Design review of the part built by this model. Coordinates are the model's own, in mm. Give positions to 0.01 mm unless a question says otherwise; leave off trailing zeros. Use CSV: the item, a comma, the result in double quotes.
from build123d import *

# Parameters (mm, degrees)
SKETCH2_W           = 3.175
SKETCH2_H           = 5.08
BOSS_EXTRUDE1_DEPTH = 3.175


with BuildPart() as part:
    # Sketch2 → Boss-Extrude1 (new body)
    with BuildSketch(Plane(origin=(0, 0, 0), x_dir=(1, 0, 0), z_dir=(0, 1, 0))):
        Polygon((-58.640729436, -170.164220965), (150.909270564, -170.164220965), (150.909270564, -134.604220965), (141.384270564, -134.604220965), (141.384270564, -129.524220965), (150.909270564, -129.524220965), (150.909270564, -93.964220965), (141.384270564, -93.964220965), (141.384270564, -88.884220965), (150.909270564, -88.884220965), (150.909270564, -43.164220965), (141.384270564, -43.164220965), (141.384270564, -38.084220965), (150.909270564, -38.084220965), (150.909270564, -2.524220965), (141.384270564, -2.524220965), (141.384270564, 2.555779035), (150.909270564, 2.555779035), (150.909270564, 39.385779035), (-58.640729436, 39.385779035), (-58.640729436, 2.555779035), (-49.115729436, 2.555779035), (-49.115729436, -2.524220965), (-58.640729436, -2.524220965), (-58.640729436, -38.084220965), (-49.115729436, -38.084220965), (-49.115729436, -43.164220965), (-58.640729436, -43.164220965), (-58.640729436, -88.884220965), (-49.115729436, -88.884220965), (-49.115729436, -93.964220965), (-58.640729436, -93.964220965), (-58.640729436, -129.524220965), (-49.115729436, -129.524220965), (-49.115729436, -134.604220965), (-58.640729436, -134.604220965), align=None)
        with Locations((-53.878229436, -162.544220965)):
            Rectangle(SKETCH2_W, SKETCH2_H, mode=Mode.SUBTRACT)
        with Locations((146.146770564, -162.544220965)):
            Rectangle(SKETCH2_W, SKETCH2_H, mode=Mode.SUBTRACT)
        with Locations((-53.878229436, -152.384220965)):
            Rectangle(SKETCH2_W, SKETCH2_H, mode=Mode.SUBTRACT)
        with Locations((-53.878229436, -142.224220965)):
            Rectangle(SKETCH2_W, SKETCH2_H, mode=Mode.SUBTRACT)
        with Locations((-53.878229436, -121.904220965)):
            Rectangle(SKETCH2_W, SKETCH2_H, mode=Mode.SUBTRACT)
        with Locations((-53.878229436, -111.744220965)):
            Rectangle(SKETCH2_W, SKETCH2_H, mode=Mode.SUBTRACT)
        with Locations((-53.878229436, -101.584220965)):
            Rectangle(SKETCH2_W, SKETCH2_H, mode=Mode.SUBTRACT)
        with Locations((-53.878229436, -81.264220965)):
            Rectangle(SKETCH2_W, SKETCH2_H, mode=Mode.SUBTRACT)
        with Locations((-53.878229436, -71.104220965)):
            Rectangle(SKETCH2_W, SKETCH2_H, mode=Mode.SUBTRACT)
        with Locations((-53.878229436, -60.944220965)):
            Rectangle(SKETCH2_W, SKETCH2_H, mode=Mode.SUBTRACT)
        with Locations((-53.878229436, -50.784220965)):
            Rectangle(SKETCH2_W, SKETCH2_H, mode=Mode.SUBTRACT)
        with Locations((-53.878229436, -30.464220965)):
            Rectangle(SKETCH2_W, SKETCH2_H, mode=Mode.SUBTRACT)
        with Locations((-53.878229436, -20.304220965)):
            Rectangle(SKETCH2_W, SKETCH2_H, mode=Mode.SUBTRACT)
        with Locations((-53.878229436, -10.144220965)):
            Rectangle(SKETCH2_W, SKETCH2_H, mode=Mode.SUBTRACT)
        with Locations((-53.878229436, 10.175779035)):
            Rectangle(SKETCH2_W, SKETCH2_H, mode=Mode.SUBTRACT)
        with Locations((-53.878229436, 20.335779035)):
            Rectangle(SKETCH2_W, SKETCH2_H, mode=Mode.SUBTRACT)
        with Locations((-53.878229436, 30.495779035)):
            Rectangle(SKETCH2_W, SKETCH2_H, mode=Mode.SUBTRACT)
        with Locations((146.146770564, 30.495779035)):
            Rectangle(SKETCH2_W, SKETCH2_H, mode=Mode.SUBTRACT)
        with Locations((146.146770564, 20.335779035)):
            Rectangle(SKETCH2_W, SKETCH2_H, mode=Mode.SUBTRACT)
        with Locations((146.146770564, 10.175779035)):
            Rectangle(SKETCH2_W, SKETCH2_H, mode=Mode.SUBTRACT)
        with Locations((146.146770564, -10.144220965)):
            Rectangle(SKETCH2_W, SKETCH2_H, mode=Mode.SUBTRACT)
        with Locations((146.146770564, -20.304220965)):
            Rectangle(SKETCH2_W, SKETCH2_H, mode=Mode.SUBTRACT)
        with Locations((146.146770564, -30.464220965)):
            Rectangle(SKETCH2_W, SKETCH2_H, mode=Mode.SUBTRACT)
        with Locations((146.146770564, -50.784220965)):
            Rectangle(SKETCH2_W, SKETCH2_H, mode=Mode.SUBTRACT)
        with Locations((146.146770564, -60.944220965)):
            Rectangle(SKETCH2_W, SKETCH2_H, mode=Mode.SUBTRACT)
        with Locations((146.146770564, -71.104220965)):
            Rectangle(SKETCH2_W, SKETCH2_H, mode=Mode.SUBTRACT)
        with Locations((146.146770564, -81.264220965)):
            Rectangle(SKETCH2_W, SKETCH2_H, mode=Mode.SUBTRACT)
        with Locations((146.146770564, -101.584220965)):
            Rectangle(SKETCH2_W, SKETCH2_H, mode=Mode.SUBTRACT)
        with Locations((146.146770564, -111.744220965)):
            Rectangle(SKETCH2_W, SKETCH2_H, mode=Mode.SUBTRACT)
        with Locations((146.146770564, -121.904220965)):
            Rectangle(SKETCH2_W, SKETCH2_H, mode=Mode.SUBTRACT)
        with Locations((146.146770564, -142.224220965)):
            Rectangle(SKETCH2_W, SKETCH2_H, mode=Mode.SUBTRACT)
        with Locations((146.146770564, -152.384220965)):
            Rectangle(SKETCH2_W, SKETCH2_H, mode=Mode.SUBTRACT)
    extrude(amount=BOSS_EXTRUDE1_DEPTH)


solid = part.part
(1) Wall thickness on line 1 along X through (y, z) = (1.85, 11): over which ranges is the line inside the solid? List them lowest first. Write a range as [from, to].
A:
line 1,"[-58.64, -55.47], [-52.29, 144.56], [147.73, 150.91]"
(2) We need section A-A on y = 2. Count the separate pieces of the cut face and the enclosed holes in it, then the cut area to 3 significant figures.
A:
separate pieces,"1"
enclosed holes,"32"
area,"43,000 mm²"
(3) Clearance check with a flat-ended pin moving along its axis: P1, Ø1, axis at y = 2.5, z = 132.5, coming from the +X side. State where the tip first meets the part, or that it passes through.
A:
P1,"x = 141.38"
